```python
from build123d import *
from OCP.BRepFilletAPI import BRepFilletAPI_MakeChamfer

# Parameters (mm, degrees)
CUT_EXTRUDE1_START  = -4
CUT_EXTRUDE1_DEPTH  = 10
BOSS_EXTRUDE1_DEPTH = 16
CHAMFER3_SIZE       = 10
CHAMFER1_SIZE       = 3
CHAMFER1_SIZE2      = 2.716212543
SKETCH4_R           = 1.75
CUT_EXTRUDE2_DEPTH  = 11
SKETCH5_R           = 1.5
CUT_EXTRUDE3_DEPTH  = 73.60961678
SKETCH6_R           = 5
CUT_EXTRUDE4_DEPTH  = 10


with BuildPart() as part:
    # Sketch1 → Revolve1 (revolve)
    with BuildSketch(Plane.XY, mode=Mode.PRIVATE) as revolve1_sk:
        Polygon((-30, 0), (-30, 3), (-18, 15), (0, 15), (0, 0), align=None)
    revolve(revolve1_sk.sketch.rotate(Axis((0, 15, 0), (0, -1, 0)), 270), axis=Axis((0, 15, 0), (0, -1, 0)))

    # Sketch2 → Cut-Extrude1 (cut)
    with BuildSketch(Plane(origin=(0, 0, 0), x_dir=(0, 0, 1), z_dir=(0.9935718556765875, -0.11320321376790697, 0)).offset(CUT_EXTRUDE1_START)):
        Polygon((7.866459251, -16.941235683), (5.5, -2), (-5.5, -2), (-7.866459251, -16.941235683), align=None)
    extrude(amount=-CUT_EXTRUDE1_DEPTH, mode=Mode.SUBTRACT)

    # Sketch3 → Boss-Extrude1 (add)
    with BuildSketch(Plane(origin=(-3.974287423, 0.452812855, 0), x_dir=(0, 0, 1), z_dir=(-0.9935718556765875, 0.11320321376790698, 0))):
        Polygon((-6.995953226, 14.641303557), (-12.539408637, 49.641303557), (12.539408637, 49.641303557), (6.995953226, 14.641303557), align=None)
    extrude(amount=-BOSS_EXTRUDE1_DEPTH)

    # Chamfer3
    chamfer3_edges = [part.edges().sort_by_distance(p)[0] for p in [
        (17.542417366, 47.963763528, 0),
    ]]
    chamfer(chamfer3_edges, length=CHAMFER3_SIZE)

    # Chamfer1: one chamfer whose edges measure the first distance from different faces: ONE call of the kernel's chamfer builder (chamfer() names one face for all edges)
    chamfer1_edges_1 = [part.edges().sort_by_distance(p)[0] for p in [
        (15.098528073, 26.514022486, 9.12012375),
        (15.098528073, 26.514022486, -9.12012375),
    ]]
    chamfer1_edges_2 = [part.edges().sort_by_distance(p)[0] for p in [
        (12.008542019, 43.561920319, -11.747486436),
        (12.008542019, 43.561920319, 11.747486436),
    ]]
    chamfer1_side_2 = [part.faces().sort_by_distance(p)[0] for p in [
        (11.909629587, 43.686270289, 0),
    ]]
    chamfer1 = BRepFilletAPI_MakeChamfer(part.part.solid().wrapped)
    for e in chamfer1_edges_1:
        chamfer1.Add(CHAMFER1_SIZE, e.wrapped)
    for e in chamfer1_edges_2:
        chamfer1.Add(CHAMFER1_SIZE, CHAMFER1_SIZE2, e.wrapped, chamfer1_side_2[0].wrapped)  # the first distance lies on this face
    add(Compound.cast(chamfer1.Shape()), mode=Mode.REPLACE)

    # Sketch4 → Cut-Extrude2 (cut)
    with BuildSketch(Plane.XZ):
        with Locations(Location((-16, 0, 0), (0, 0, 270))):
            Circle(SKETCH4_R)
        with Locations(Location((16, 0, 0), (0, 0, 270))):
            Circle(SKETCH4_R)
    extrude(amount=-CUT_EXTRUDE2_DEPTH, mode=Mode.SUBTRACT)

    # Sketch5 → Cut-Extrude3 (cut, through all)
    with BuildSketch(Plane(origin=(11.922862268, -1.358438565, 0), x_dir=(0, 0, -1), z_dir=(0.9935718556765875, -0.11320321376790698, 0))):
        with Locations(Location((0, 41.46427329, 0), (0, 0, 90))):
            Circle(SKETCH5_R)
    extrude(amount=-CUT_EXTRUDE3_DEPTH, mode=Mode.SUBTRACT)

    # Sketch6 → Cut-Extrude4 (cut)
    with BuildSketch(Plane(origin=(11.922862268, -1.358438565, 0), x_dir=(0, 0, -1), z_dir=(0.9935718556765875, -0.11320321376790698, 0))):
        with Locations(Location((0, 41.46427329, 0), (0, 0, 90))):
            Circle(SKETCH6_R)
    extrude(amount=-CUT_EXTRUDE4_DEPTH, mode=Mode.SUBTRACT)


solid = part.part
```
Build history of the part. All positions in model axes, mm. A direction names the side the tool comes from. Coordinates: 2 decimals unless noted, no trailing zeros. Write each loop counter-clockwise with the first axis right and the second up, starting at its lowest first coordinate (ties: lowest second). Pieces come first, ordered by that corner, then holes.
1. Band-saw the part on C-C, the plane y = 18.5. Give the cut face in (x, z), and give its area (3 significant figures).
Answer block:
outline: (-1.92, -7.55) - (11.17, -7.79) - (14.19, -4.81) - (14.19, 4.81) - (11.17, 7.79) - (-1.92, 7.55) - close
area: 239 mm2
2. Drop flat-ended pins along their axis: pin 1 (3 mm diameter, centred on x = 16, z = 0, fed in from -Y); pin 2 (1 mm diameter, centred on y = 13, z = -10, fed in from +X); pin 3 (3 mm diameter, centred on x = -16, z = 0, fed in from +Y). Give the stop position or say it passes through.
Answer block:
pin 1: stops at y = 11
pin 2: stops at x = 17.96
pin 3: stops at y = 15
3. Band-saw the part on D-D, the plane y = 26. Give the cut face in (x, z), and give its area (3 significant figures).
Answer block:
outline: (-1.06, -8.75) - (12.02, -8.98) - (15.04, -6) - (15.04, 6) - (12.02, 8.98) - (-1.06, 8.75) - close
area: 277 mm2
4. Pull direction Y, two halves, no side cores. Call faces 5 (the flat face through (13.586, 26.301, -7.519)), 6 (the flat face through (-0.414, 31.698, 0.176)), 7 (the flat face through (16, 11, 0)): released by +Y, released by -Y, zero draft, split by the parting line, or undercut.
Answer block:
face 5: undercut
face 6: released by +Y
face 7: released by -Y
5. 3-axis set-ups, long thin cutter, end or side, ignore diameter. For faces 1 (the flat face through (13.58, 26.62, 7.61)), 2 (the cylindrical face through (-14.265, 5.423, 0.228)), 3 (the flat face through (-13.04, 9.21, -0.1)), 4 (the flat face through (15.117, 26.675, 0.111)): which of +Z, -Z, +X, -X, +Y, -Y reach the whole face in a straight line?
Answer block:
face 1: +Z, +X
face 2: -Y
face 3: none
face 4: +Z, -Z, +X
6. Band-saw the part on A-A, the plane y = 9. Give the cut face in (x, z), and give its area (3 significant figures).
Answer block:
outline: circle Ø48 at (0, 0); hole circle Ø3.5 at (-16, 0); hole (-13.07, -6.37) - (-3, -6.55) - (-3, 6.55) - (-13.07, 6.37) - close; hole circle Ø3.5 at (16, 0)
area: 1,660 mm2
7. Band-saw the part on B-B, the plane z = 0. Give the cut face in (x, y).
Answer block:
outline: (-30, 0) - (-17.75, 0) - (-17.75, 11) - (-14.25, 11) - (-14.25, 0) - (14.25, 0) - (14.25, 11) - (17.75, 11) - (17.75, 0) - (30, 0) - (30, 3) - (18, 15) - (13.79, 15) - (16.05, 34.87) - (6.12, 36) - (6.51, 39.48) - (0.55, 40.16) - (-3.75, 2.44) - (-13.68, 3.57) - (-12.38, 15) - (-18, 15) - (-30, 3) - close; (0.89, 43.14) - (6.85, 42.46) - (7.25, 45.94) - (10.4, 45.58) - (7.61, 49.1) - (1.65, 49.78) - close
8. Drill centre lines: probe 1 along X at (y, z) = (6.75, 0); probe 2 along Y at (x, z) = (2, -23); probe 3 along Z at (x, y) = (14, 3). Where is each one in solid material? Low to high.
Answer block:
probe 1: x = -26.25 to -17.75, -14.25 to -13.32, -3.26 to 14.25, 17.75 to 26.25
probe 2: y = 0 to 9.91
probe 3: z = -26.53 to 26.53
